Design review of the part built by this model. Coordinates are the model's own, in mm. Face numbers are marked on the shaded views. Coordinates: 2 decimals unless noted, no trailing zeros. Write each loop counter-clockwise with the first axis right and the second up, starting at its lowest first coordinate (ties: lowest second). Pieces come first, ordered by that corner, then holes.
Q1. Add section A-A, the plane x = -22. Give the boundary of the cut face in (y, z).
Q2. Add section D-D, the plane y = -175.5. Give the boundary of the cut face in (x, z).
Q3. Add section C-C, the plane x = 48. Give the boundary of the cut face in (y, z).
Q4. Clearance check with flat-ended pins moving along their axes: pin 1 Ø3 at (y, z) = (-115.5, 12.5) entering from -X; pin 2 Ø1 at (y, z) = (-24, 15.5) entering from +X; pin 3 Ø6 at (x, z) = (-50, 19.5) entering from -Y. State where each tip first meets the part, or that it passes through.
Q5. Add section B-B, the plane z = 17.5. Give the boundary of the cut face in (x, y).
Q6. To check wall thickness, follow probe 1 along Y at (x, z) = (-8.5, 10.25); probe 2 along X at (y, z) = (-200.5, 26.75); probe 3 along X at (y, z) = (-151, 16.25). State the ranges of each line that lie inside material, in increasing order.
Q7. The part is to be moulded in two halves that separate along X. For the marked faces 1, 2 and 3, say which applies: +X half, -X half, draft (parallel to the pull), parting line (faces both ways), or undercut.
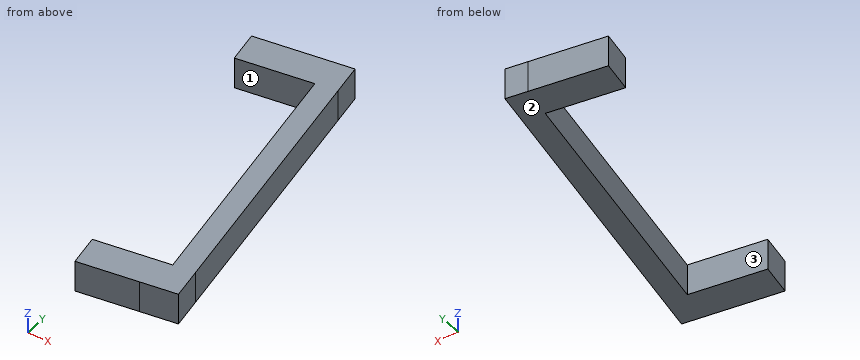
Autodesk Inventor part; units mm, degrees
ref_plane "YZ Plane" through (0, 0, 0) normal (1, 0, 0) x (0, 1, 0)
ref_plane "XZ Plane" through (0, 0, 0) normal (0, 1, 0) x (-1, 0, 0)
ref_plane "XY Plane" through (0, 0, 0) normal (0, 0, 1) x (1, 0, 0)
sketch "Sketch1" plane through (0, 0, 0) normal (0, 0, 1) x (1, 0, 0)
  arc A0 (5.5018, -3.1706) -> (4.1426, 4.8126) centre (0, 0) ccw
  line L0 (-0.2789, 17.1872) -> (4.1426, 4.8126)
  arc A1 (-0.2789, 17.1872) -> (-5.4243, 16.3111) centre (-2.7743, 16.2955) ccw
  line L1 (-5.5018, 3.1706) -> (-5.4243, 16.3111)
  arc A2 (-5.5018, 3.1706) -> (-4.1426, -4.8126) centre (0, 0) ccw
  line L2 (-4.1426, -4.8126) -> (0.2789, -17.1872)
  arc A3 (0.2789, -17.1872) -> (5.4243, -16.3111) centre (2.7743, -16.2955) ccw
  line L3 (5.4243, -16.3111) -> (5.5018, -3.1706)
  circle A4 centre (1.7673, -10.3806) radius 0.5
  circle A5 centre (1.2638, -7.4232) radius 0.5
  circle A6 centre (0, 0) radius 4.375
  circle A7 centre (-2.2708, 13.3381) radius 0.5
  circle A8 centre (-1.7673, 10.3806) radius 0.5
  circle A9 centre (-1.2638, 7.4232) radius 0.5
  circle A10 centre (-2.7743, 16.2955) radius 0.5
  circle A11 centre (2.2708, -13.3381) radius 0.5
  circle A12 centre (2.7743, -16.2955) radius 0.5
  line L4 (0, 0) -> (2.7743, -16.2955)
  line L5 (0, 0) -> (47.7501, -296.1755)
  line L6 (0, 0) -> (23.8751, -148.0877)
  line L7 (-9.8725, -1.5917) -> (37.8776, -297.7672)
  line L8 (37.8776, -297.7672) -> (57.6226, -294.5838)
  line L9 (57.6226, -294.5838) -> (9.8725, 1.5917)
  line L10 (9.8725, 1.5917) -> (-9.8725, -1.5917)
  line L11 (-9.8725, -1.5917) -> (57.6226, -294.5838) construction
  line L12 (37.8776, -297.7672) -> (9.8725, 1.5917) construction
  circle A13 centre (0, 0) radius 25
  point P0 (13.5195, -21.0291)
  point P1 (-6.2255, -24.2124)
  dimension "d0" = 300
  dimension "d1" = 150
  dimension "d2" = 20
  dimension "d3" = 50
extrude "Extrusion1" add sketch "Sketch1" along normal blind 30 contours L3 A3 L5 A12 L4 A11 A4 A5 A6 L10 A0 | A0 L10 L9 A13 L5 A3 L3 | L10 A6 A2 L1 A1 L0 A0 | A0 L0 A1 L1 A2 L10 L7 A13 L9 | L10 A6 | A6 L4 L10 | L5 A13 L7 L10 A2 L2 A3 | A3 L2 A2 L10 A6 L5 A5 A4 A11 A12 | L9 L8 L5 A13 | L10 L5 A6 | L4 A6 L5 | L5 A12 | A12 L5 | L5 L8 L7 A13 | L4 A5 L5 A6 | L5 A11 L4 A12 | L4 A5 L5 | A5 L4 | L5 A5 | L5 A11 L4 | A11 L5 | L4 A4 L5 A5 | L4 A11 | L5 A4 L4 A11 | L4 A4 L5 | A4 L4 | L5 A4 | A7 | A8 | A9 | A10
sketch "Sketch2" plane through (37.8776, -297.7672, 0) normal (-0.9872517, -0.159167, 0) x (0, 0, 1)
  line L0 (30, 277.0871) -> (30, 0)
  line L1 (30, 0) -> (0, 0)
  line L2 (0, 0) -> (0, 30)
  line L3 (0, 30) -> (30, 30)
  line L4 (30, 30) -> (30, 0)
  point P0 (0, 300)
  point P1 (30, 30)
  dimension "d6" = 30
  dimension "d7" = 30
extrude "Extrusion2" add sketch "Sketch2" along normal blind 70
sketch "Sketch4" plane through (0, 0, 30) normal (0, 0, 1) x (1, 0, 0)
  line L0 (-6.2255, -24.2124) -> (33.1026, -268.1496)
  line L1 (33.1026, -268.1496) -> (-36.005, -279.2913)
  line L2 (-31.23, -308.9089) -> (-36.005, -279.2913)
  line L3 (57.6226, -294.5838) -> (-31.23, -308.9089)
  line L4 (57.6226, -294.5838) -> (13.5195, -21.0291)
  arc A0 (13.5195, -21.0291) -> (-6.2255, -24.2124) centre (0, 0) ccw
  arc A1 (13.5195, -21.0291) -> (-6.2255, -24.2124) centre (0, 0) ccw
  circle A2 centre (0, 0) radius 25
  point P0 (13.5195, -21.0291)
extrude "Extrusion4" cut sketch "Sketch4" against normal through all contours A0 A2
sketch "Sketch5" plane through (0, 0, 30) normal (0, 0, 1) x (1, 0, 0)
  arc A0 (-6.2255, -24.2124) -> (13.5195, -21.0291) centre (0, 0) ccw
  line L0 (-6.2255, -24.2124) -> (33.1026, -268.1496)
  line L1 (33.1026, -268.1496) -> (-36.005, -279.2913)
  line L2 (-31.23, -308.9089) -> (-36.005, -279.2913)
  line L3 (57.6226, -294.5838) -> (-31.23, -308.9089)
  line L4 (57.6226, -294.5838) -> (13.5195, -21.0291)
  line L5 (-6.2255, -24.2124) -> (33.1026, -268.1496)
  line L6 (-6.2255, -24.2124) -> (13.5195, -21.0291)
extrude "Extrusion5" add sketch "Sketch5" against normal up to surface (30 mm away) contours L6 A0
ref_plane "Work Plane2" through (33.1836, -142.9977, 0) normal (0.159167, -0.9872517, 0) x (0.9872517, 0.159167, 0)
ref_plane "Work Plane1" through (52.8476, -264.9663, 0) normal (0.159167, -0.9872517, 0) x (0.9872517, 0.159167, 0)
mirror "Mirror1" about plane through (33.1836, -142.9977, 0) normal (0.159167, -0.9872517, 0) of "Extrusion2"
mirror "Mirror2" about plane through (33.1836, -142.9977, 0) normal (0.159167, -0.9872517, 0) of "Extrusion1"
sketch "Sketch6" plane through (0, 0, 30) normal (0, 0, 1) x (1, 0, 0)
  line L0 (33.1026, -268.1496) -> (-36.005, -279.2913)
  line L1 (-31.23, -308.9089) -> (-36.005, -279.2913)
  line L2 (24.0813, -299.9914) -> (-31.23, -308.9089)
  arc A0 (24.0813, -299.9914) -> (52.8476, -264.9663) centre (46.6221, -289.1787) ccw
  line L3 (52.8476, -264.9663) -> (8.7445, 8.5884)
  line L4 (-80.1082, -5.7366) -> (8.7445, 8.5884)
  line L5 (-80.1082, -5.7366) -> (-75.3332, -35.3541)
  line L6 (-6.2255, -24.2124) -> (-75.3332, -35.3541)
  line L7 (-6.2255, -24.2124) -> (33.1026, -268.1496)
  line L8 (-36.005, -279.2913) -> (-31.23, -308.9089)
  line L9 (-36.005, -279.2913) -> (52.8476, -264.9663)
  line L10 (24.0813, -299.9914) -> (-31.23, -308.9089)
  line L11 (-31.23, -308.9089) -> (57.6226, -294.5838)
  line L12 (57.6226, -294.5838) -> (52.8476, -264.9663)
  point P0 (0, 0)
extrude "Extrusion6" cut sketch "Sketch6" against normal through all contours A0 L11 L12
sketch "Sketch7" plane through (0, 0, 30) normal (0, 0, 1) x (1, 0, 0)
  point P0 (0, 0)
sketch "Sketch8" plane through (0, 0, 30) normal (0, 0, 1) x (1, 0, 0)
  line L0 (-31.23, -308.9089) -> (-36.005, -279.2913)
  line L1 (-6.2255, -24.2124) -> (33.1026, -268.1496)
  line L2 (-36.005, -279.2913) -> (33.1026, -268.1496)
  point P0 (0, 0)
properties part number "arm" material "PET Plastic"
Here are the results:
1. outline: (-307.42, 0) - (-277.03, 0) - (-277.03, 30) - (-307.42, 30) - close; (-26.76, 0) - (3.63, 0) - (3.63, 30) - (-26.76, 30) - close
2. outline: (18.17, 0) - (38.42, 0) - (38.42, 30) - (18.17, 30) - close
3. outline: (-296.14, 0) - (-234.9, 0) - (-234.9, 30) - (-296.14, 30) - close
4. pin 1: stops at x = 8.25
4. pin 2: stops at x = 14.08
4. pin 3: stops at y = -31.75
5. outline: (-80.11, -5.74) - (-75.33, -35.35) - (-6.23, -24.21) - (33.1, -268.15) - (-36.01, -279.29) - (-31.23, -308.91) - (24.08, -299.99) - (57.62, -294.58) - (8.74, 8.59) - (-11, 5.41) - close
6. probe 1: y = -305.24 to -274.86, -24.58 to 5.81
6. probe 2: x = 22.2 to 42.45
6. probe 3: x = 14.22 to 34.47
7. face 1: undercut
7. face 2: draft
7. face 3: -X half
